Model file for the job. Use its own axes, mm. A direction names the side the tool comes from. Round coordinates to 2 decimals unless told otherwise and drop trailing zeros. Loops run counter-clockwise (first coordinate to the right, second up) from the corner with the lowest first, then second, coordinate; pieces in that order, holes last. Notation, with made-up numbers: (-14, 41.5) -> (31, 41.5) arc R29 ccw to (31, 71.5) -> close; hole circle Ø8 at (-6, -22.75). An arc over 180 degrees is marked (long way). Use a Markdown table: item, result.
Autodesk Inventor part; units mm, degrees
ref_plane "YZ Plane" through (0, 0, 0) normal (1, 0, 0) x (0, 1, 0)
ref_plane "XZ Plane" through (0, 0, 0) normal (0, 1, 0) x (-1, 0, 0)
ref_plane "XY Plane" through (0, 0, 0) normal (0, 0, 1) x (1, 0, 0)
sketch "Skizze1" plane through (0, 0, 0) normal (0, 0, 1) x (1, 0, 0)
  line L0 (-29.61, 0) -> (29.61, 0)
  line L1 (0, -29.61) -> (0, 29.61)
  line L2 (21.15, -21.15) -> (-21.15, -21.15)
  line L3 (-21.15, -21.15) -> (-21.15, 21.15)
  line L4 (-21.15, 21.15) -> (21.15, 21.15)
  line L5 (21.15, 21.15) -> (21.15, -21.15)
  line L6 (21.15, -21.15) -> (-21.15, 21.15) construction
  line L7 (-21.15, -21.15) -> (21.15, 21.15) construction
  point P0 (0, 0)
  dimension "d0" = 42.3
  dimension "d1" = 42.3
extrude "Extrusion1" add sketch "Skizze1" along normal blind 60
sketch "Skizze2" plane through (0, 0, 60) normal (0, 0, 1) x (1, 0, 0)
  circle A0 centre (0, 0) radius 11
  dimension "d4" = 22
extrude "Extrusion2" add sketch "Skizze2" along normal blind 2
sketch "Skizze3" plane through (0, 0, 62) normal (0, 0, 1) x (1, 0, 0)
  circle A0 centre (0, 0) radius 2.5
  dimension "d7" = 5
extrude "Extrusion3" add sketch "Skizze3" along normal blind 22
sketch "Skizze4" plane through (0, 0, 60) normal (0, 0, 1) x (1, 0, 0)
  circle A0 centre (0, 0) radius 11
  line L0 (21.15, 21.15) -> (-21.15, 21.15)
  line L1 (-21.15, 21.15) -> (-21.15, -21.15)
  line L2 (-21.15, -21.15) -> (21.15, -21.15)
  line L3 (21.15, -21.15) -> (21.15, 21.15)
  line L4 (15.5, -15.5) -> (-15.5, -15.5)
  line L5 (-15.5, -15.5) -> (-15.5, 15.5)
  line L6 (-15.5, 15.5) -> (15.5, 15.5)
  line L7 (15.5, 15.5) -> (15.5, -15.5)
  line L8 (15.5, -15.5) -> (-15.5, 15.5) construction
  line L9 (-15.5, -15.5) -> (15.5, 15.5) construction
  dimension "d10" = 31
  dimension "d11" = 31
hole "Bohrung1" at (-15.5, 15.5, 60) at (15.5, 15.5, 60) at (15.5, -15.5, 60) at (-15.5, -15.5, 60) direction (0, 0, -1) diameter 2.459 depth 8.8 tip angle 118
chamfer "Fasen1" distance 5 angle 45 4 edges at (21.15, -21.15, 30) (21.15, 21.15, 30) (-21.15, 21.15, 30) (-21.15, -21.15, 30)
equation "\"d1\" = d0"
equation "\"d11\" = d10"
properties part number "Motor ST4118D1804-A"
Q1. Band-saw the part on D-D, the plane x = 4.5. Give the cut face in (y, z), plus the area to 3 significant figures.
Results list:
| item | result |
|---|---|
| outline | (-21.15, 0) -> (21.15, 0) -> (21.15, 60) -> (10.04, 60) -> (10.04, 62) -> (-10.04, 62) -> (-10.04, 60) -> (-21.15, 60) -> close |
| area | 2,580 mm² |
Q2. Pull direction X, two halves, no side cores. Call faces 1 (the face through (-2.38, 10.74, 60.99)), 2 (the face through (15.131, -16.673, 55.538)), 3 (the face through (18.7, -18.6, 30.4)), 4 (the face through (14.463, 14.839, 55.538)): released by +X, released by -X, zero draft, split by the parting line, or undercut.
Results list:
| item | result |
|---|---|
| face 1 | split by the parting line |
| face 2 | undercut |
| face 3 | released by +X |
| face 4 | undercut |
Q3. Tool access for faces 5 (the face through (-0.54, 2.44, 72.85)), 6 (the face through (0, -21.15, 30)): list every direction of +Z, -Z, +X, -X, +Y, -Y with a clear straight run to the whole face (end or side of a thin tool).
Results list:
| item | result |
|---|---|
| face 5 | +Z |
| face 6 | +Z, -Z, +X, -X, -Y |
Q4. Drill centre lines: L1, parallel to Y at x = 15.5, z = 55.5; L2, parallel to X at y = -14.5, z = 53. Where is each one in solid material? Low to high. Write a range as from..to.
Results list:
| item | result |
|---|---|
| L1 | y = -21.15..-16.73, -14.27..14.27, 16.73..21.15 |
| L2 | x = -21.15..-16.22, -14.78..14.78, 16.22..21.15 |
Q5. Band-saw the part on B-B, the plane x = 0. Give the cut face in (y, z).
Results list:
| item | result |
|---|---|
| outline | (-21.15, 0) -> (21.15, 0) -> (21.15, 60) -> (11, 60) -> (11, 62) -> (2.5, 62) -> (2.5, 84) -> (-2.5, 84) -> (-2.5, 62) -> (-11, 62) -> (-11, 60) -> (-21.15, 60) -> close |
Q6. Flat gauge pins, fed straight in: pin 1 (2 mm diameter, centred on x = -11, y = 15, fed in from +Z); pin 2 (2 mm diameter, centred on x = -15.5, y = -15.5, fed in from +Z); pin 3 (6 mm diameter, centred on x = -9.5, y = 10, fed in from +Z). Where does each tip first touch, or does it go through?
Results list:
| item | result |
|---|---|
| pin 1 | stops at z = 60 |
| pin 2 | stops at z = 51.06 |
| pin 3 | stops at z = 62 |
Q7. Band-saw the part on A-A, the plane z = 41.5. Give the cut face in (x, y).
Results list:
| item | result |
|---|---|
| outline | (-21.15, -16.15) -> (-16.15, -21.15) -> (16.15, -21.15) -> (21.15, -16.15) -> (21.15, 16.15) -> (16.15, 21.15) -> (-16.15, 21.15) -> (-21.15, 16.15) -> close |
